```python
from build123d import *

# Parameters (mm, degrees)
F_19_64_0_29688_DIAMETER_HOLE1_D = 7.540752
CHAMFER1_SIZE                    = 0.79375


with BuildPart() as part:
    # Sketch1 → Revolve1 (revolve)
    with BuildSketch(Plane(origin=(0, 0, 0), x_dir=(0, 0, -1), z_dir=(1, 0, 0))):
        Polygon((0, -4.460875), (-7.9375, -4.460875), (-7.9375, -2.238375), (-5.953125, -2.238375), (-5.953125, 2.930525), (-5.6261, 2.930525), (-5.6261, 3.667125), (-5.953125, 3.667125), (-5.953125, 4.460875), (0, 4.460875), align=None)
    revolve(axis=Axis((0, 0, 0), (0, 1, 0)))

    # 19/64 (0.29688) Diameter Hole1 (through all)
    with Locations(Plane(origin=(0, 4.460875, 0), x_dir=(1, 0, 0), z_dir=(0, 1, 0))):
        with Locations((0, 0)):
            Hole(F_19_64_0_29688_DIAMETER_HOLE1_D / 2)

    # Chamfer1
    chamfer1_edges = [part.edges().sort_by_distance(p)[0] for p in [
        (3.770376, -4.460875, 0),
    ]]
    chamfer(chamfer1_edges, length=CHAMFER1_SIZE)


solid = part.part
```
The model under review builds one solid part; all positions refer to its coordinate system, in mm. A direction names the side the tool comes from. Coordinates: 2 decimals unless noted, no trailing zeros. Write each loop counter-clockwise with the first axis right and the second up, starting at its lowest first coordinate (ties: lowest second). Pieces come first, ordered by that corner, then holes. Notation, with made-up numbers: (71, 35) -> (109, 35) arc R26 ccw to (109, 74) -> close; hole circle Ø1 at (74, 63.5). An arc over 180 degrees is marked (long way). One line per item, written item: value. Start each with the question number.
Q1. Add section D-D, the plane x = -5.25. Give the boundary of the cut face in (y, z).
Q2. For faces 1 (the face through (6, -2.238, -2)), 2 (the face through (3.767, 0.34, -0.166)), list the 3-axis set-ups (+Z, -Z, +X, -X, +Y, -Y) from which the entire face can be reached by the end or side of a thin tool; tool diameter is ignored.
Q3. Add section A-A, the plane x = 0. Give the boundary of the cut face in (y, z).
Q4. Add section C-C, the plane y = -0.5. Give the boundary of the cut face in (x, z).
Q5. To check wall thickness, follow probe 1 along Y at (x, z) = (-5, 2.75); probe 2 along X at (y, z) = (0, 0); probe 3 along Z at (x, y) = (5.25, -4). State the ranges of each line that lie inside material, in increasing order.
Q6. Clearance check with flat-ended pins moving along their axes: P1, Ø1.5, axis at x = 4.5, y = -2, coming from the -Z side; P2, Ø1.5, axis at x = -3, y = 1.5, coming from the +Z side; P3, Ø4, axis at x = 4, y = 0, coming from the -Z side; P4, Ø6, axis at x = 1, z = 1.5, coming from the +Y side. State where each tip first meets the part, or that it passes through.
Q7. The part is to be moulded in two halves that separate along Y. For faces 3 (the face through (5.58, 3.3, -0.73)), 4 (the face through (-7.75, -3.33, -1.72)), 5 (the face through (-4, 4.461, 0)), 6 (the face through (-3.4, -4.461, -3.4)), say which applies: +Y half, -Y half, draft (parallel to the pull), parting line (faces both ways), or undercut.
Q8. Add section B-B, the plane z = 0. Give the boundary of the cut face in (x, y), then the cut area to 3 significant figures.
Response:
1. outline: (-4.46, -5.95) -> (-2.24, -5.95) -> (-2.24, -2.81) -> (2.93, -2.81) -> (2.93, -2.02) -> (3.67, -2.02) -> (3.67, -2.81) -> (4.46, -2.81) -> (4.46, 2.81) -> (3.67, 2.81) -> (3.67, 2.02) -> (2.93, 2.02) -> (2.93, 2.81) -> (-2.24, 2.81) -> (-2.24, 5.95) -> (-4.46, 5.95) -> close
2. face 1: +Y
2. face 2: +Y, -Y
3. outline: (-4.46, -7.94) -> (-2.24, -7.94) -> (-2.24, -5.95) -> (2.93, -5.95) -> (2.93, -5.63) -> (3.67, -5.63) -> (3.67, -5.95) -> (4.46, -5.95) -> (4.46, -3.77) -> (-3.67, -3.77) -> (-4.46, -4.56) -> close; (-4.46, 4.56) -> (-3.67, 3.77) -> (4.46, 3.77) -> (4.46, 5.95) -> (3.67, 5.95) -> (3.67, 5.63) -> (2.93, 5.63) -> (2.93, 5.95) -> (-2.24, 5.95) -> (-2.24, 7.94) -> (-4.46, 7.94) -> close
4. outline: circle Ø11.91 at (0, 0); hole circle Ø7.54 at (0, 0)
5. probe 1: -4.46 to 2.93, 3.67 to 4.46
5. probe 2: -5.95 to -3.77, 3.77 to 5.95
5. probe 3: -5.95 to 5.95
6. P1: z = -6.97
6. P2: z = 5.51
6. P3: z = -5.61
6. P4: y = 4.46
7. face 3: undercut
7. face 4: draft
7. face 5: +Y half
7. face 6: -Y half
8. outline: (-7.94, -4.46) -> (-4.56, -4.46) -> (-3.77, -3.67) -> (-3.77, 4.46) -> (-5.95, 4.46) -> (-5.95, 3.67) -> (-5.63, 3.67) -> (-5.63, 2.93) -> (-5.95, 2.93) -> (-5.95, -2.24) -> (-7.94, -2.24) -> close; (3.77, -3.67) -> (4.56, -4.46) -> (7.94, -4.46) -> (7.94, -2.24) -> (5.95, -2.24) -> (5.95, 2.93) -> (5.63, 2.93) -> (5.63, 3.67) -> (5.95, 3.67) -> (5.95, 4.46) -> (3.77, 4.46) -> close
8. area: 46.7 mm²
